```python
from build123d import *

# Parameters (mm, degrees)
CROQUIS1_W              = 244
CROQUIS1_H              = 195
SALIENTE_EXTRUIR1_DEPTH = 15


with BuildPart() as part:
    # Croquis1 → Saliente-Extruir1 (new body)
    with BuildSketch(Plane.YZ):
        with Locations((122, 97.5)):
            Rectangle(CROQUIS1_W, CROQUIS1_H)
        Polygon((163, 22.5), (136.5, 22.5), (129.831375645, 38.218900266), (129.5, 39), (129.831375684, 39.781099827), (136.5, 55.5), (163, 55.5), (169.668624522, 39.78109934), (170, 39), (169.668624483, 38.218900567), align=None, mode=Mode.SUBTRACT)
        with BuildLine():
            Line((189, 82.25), (189, 111.75))
            ThreePointArc((189, 111.75), (205.25, 128), (221.5, 111.75))
            Line((221.5, 111.75), (221.5, 82.25))
            ThreePointArc((221.5, 82.25), (205.25, 66), (189, 82.25))
        make_face(mode=Mode.SUBTRACT)
    extrude(amount=SALIENTE_EXTRUIR1_DEPTH)


solid = part.part
```
Check sheet for the modelled part. Datum: model origin and axes. Units: mm. A direction names the side the tool comes from. Round coordinates to 2 decimals unless told otherwise and drop trailing zeros. Order: outer loops, then holes, each group sorted by start corner. A loop starts at its lowest first (then second) coordinate and runs counter-clockwise, first axis right, second up.
1) Tool access check on faces 5 (the flat face through (7, 120, 195)), 6 (the flat face through (7, 221.5, 97)). Record the directions out of +Z, -Z, +X, -X, +Y, -Y that give a thin tool (end or side, any length) a straight path to the whole face; none if there is none.
2) Section check A-A (x = 10.75). Record the boundary of the cut face in (y, z), and give its area (3 significant figures).
3) Scan lines: line 1 (Z direction, x = 7.75, y = 144.5); line 2 (Z direction, x = 14, y = 205); line 3 (Y direction, x = 1, z = 80). Record each from-to range of solid material in increasing order.
4) Mould release check, pull along Z, two halves, no side actions. Record for faces 1 (the flat face through (7, 150, 22.5)), 2 (the flat face through (15, 120, 99)), 3 (the flat face through (7, 120, 0)), 4 (the cylindrical face through (7.395, 205.607, 66.004)): +Z half, -Z half, draft (parallel to the pull), parting line (faces both ways), or undercut.
5) Section check C-C (z = 97). Record the boundary of the cut face in (x, y), and give its area (3 significant figures).
6) Go/stop test with a flat-tipped pin: pin 1 Ø10 at (y, z) = (169, 34) entering from -X. Record where the tip stops, or that it passes through.
7) Section check B-B (y = 205.25). Record the boundary of the cut face in (x, z).
Result:
1. face 5: +Z, +X, -X, +Y, -Y
1. face 6: +X, -X
2. outline: (0, 0) - (244, 0) - (244, 195) - (0, 195) - close; hole (129.5, 39) - (136.5, 22.5) - (163, 22.5) - (170, 39) - (163, 55.5) - (136.5, 55.5) - close; hole (189, 82.25) arc R16.25 ccw to (221.5, 82.25) - (221.5, 111.75) arc R16.25 ccw to (189, 111.75) - close
2. area: 44,700 mm2
3. line 1: z = 0 to 22.5, 55.5 to 195
3. line 2: z = 0 to 66, 128 to 195
3. line 3: y = 0 to 189.16, 221.34 to 244
4. face 1: undercut
4. face 2: draft
4. face 3: -Z half
4. face 4: undercut
5. outline: (0, 0) - (15, 0) - (15, 189) - (0, 189) - close; (0, 221.5) - (15, 221.5) - (15, 244) - (0, 244) - close
5. area: 3,170 mm2
6. pin 1: stops at x = 0
7. outline: (0, 0) - (15, 0) - (15, 66) - (0, 66) - close; (0, 128) - (15, 128) - (15, 195) - (0, 195) - close
